Could you check a few things on this drawing? It's one solid part, dimensions in mm from its lowest x, y, z. A direction names the side the tool comes from. Give positions to 0.01 mm unless a question says otherwise; leave off trailing zeros. Order: outer loops, then holes, each group sorted by start corner. A loop starts at its lowest first (then second) coordinate and runs counter-clockwise, first axis right, second up.
(1) On a 3-axis mill with a long thin cutter (end or side, diameter ignored), from which of +Z, -Z, +X, -X, +Y, -Y can I reach the whole of each face in a straight line? I mean the marked faces 1, 2 and 3. Say none if no direction works.
(2) Imagine slicing it at A-A, the plane z = 21.5. Write out the boundary of the cut face in (x, y), then the cut area to 3 significant figures.
(3) If I drill on probe 1 along Y at (x, z) = (42.5, 28); probe 2 along Z at (x, y) = (12.5, 59); probe 3 along Z at (x, y) = (51, 43), over which ranges is the centre line in solid material (lowest first)?
(4) Will these pins go through, and if not, where does the flat tip stop? pin 1 (2 mm diameter, centred on x = 68.5, z = 184.5, fed in from -Y); pin 2 (12 mm diameter, centred on x = 24.5, y = 15.5, fed in from -Z); pin 3 (12 mm diameter, centred on x = 15.5, z = 41, fed in from +Y).
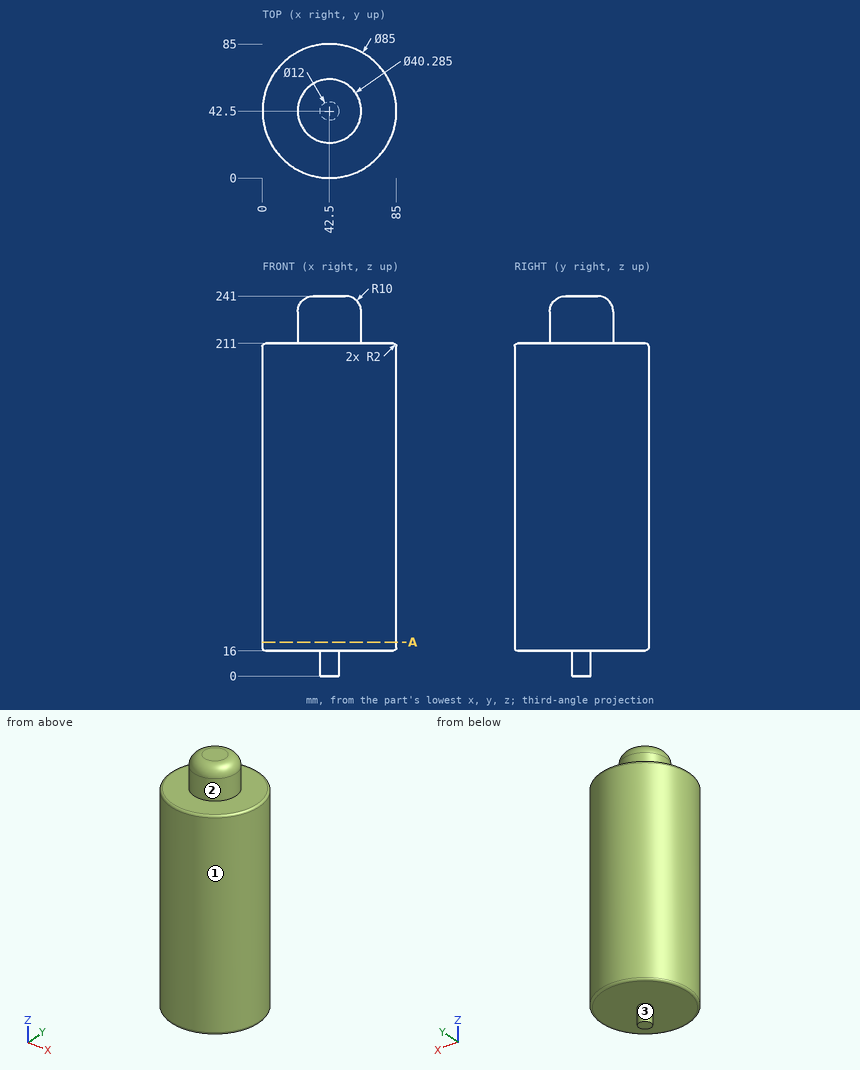
Answer block:
1. face 1: +Z, -Z
1. face 2: +Z
1. face 3: -Z
2. outline: circle Ø85 at (42.5, 42.5)
2. area: 5,670 mm2
3. probe 1: y = 0 to 85
3. probe 2: z = 16 to 211
3. probe 3: z = 16 to 241
4. pin 1: stops at y = 8.13
4. pin 2: stops at z = 16
4. pin 3: stops at y = 79.45
